```python
from build123d import *

# Parameters (mm, degrees)
SKETCH1_W           = 20
SKETCH1_H           = 20
BOSS_EXTRUDE1_DEPTH = 20
CUT_EXTRUDE1_DEPTH  = 20
CUT_EXTRUDE2_DEPTH  = 20
CUT_EXTRUDE3_DEPTH  = 20
CUT_EXTRUDE4_DEPTH  = 20


with BuildPart() as part:
    # Sketch1 → Boss-Extrude1 (new body)
    with BuildSketch(Plane.XY):
        with Locations((10, 10)):
            Rectangle(SKETCH1_W, SKETCH1_H)
    extrude(amount=BOSS_EXTRUDE1_DEPTH)

    # Sketch2 → Cut-Extrude1 (cut)
    with BuildSketch(Plane(origin=(0, 20, 0), x_dir=(1, 0, 0), z_dir=(0, 1, 0))):
        Polygon((20, 0), (10, 0), (20, -10), align=None)
    extrude(amount=-CUT_EXTRUDE1_DEPTH, mode=Mode.SUBTRACT)

    # Sketch3 → Cut-Extrude2 (cut)
    with BuildSketch(Plane(origin=(0, 20, 0), x_dir=(1, 0, 0), z_dir=(0, 1, 0))):
        Polygon((20, -20), (20, -10), (10, -20), align=None)
    extrude(amount=-CUT_EXTRUDE2_DEPTH, mode=Mode.SUBTRACT)

    # Sketch4 → Cut-Extrude3 (cut)
    with BuildSketch(Plane(origin=(0, 20, 0), x_dir=(1, 0, 0), z_dir=(0, 1, 0))):
        Polygon((0, 0), (10, 0), (0, -10), align=None)
    extrude(amount=-CUT_EXTRUDE3_DEPTH, mode=Mode.SUBTRACT)

    # Sketch5 → Cut-Extrude4 (cut)
    with BuildSketch(Plane(origin=(0, 20, 0), x_dir=(1, 0, 0), z_dir=(0, 1, 0))):
        Polygon((0, -20), (0, -10), (10, -20), align=None)
    extrude(amount=-CUT_EXTRUDE4_DEPTH, mode=Mode.SUBTRACT)


solid = part.part
```
Input: part model. Units: mm. Frame: model coordinates. Coordinates: 2 decimals unless noted, no trailing zeros. Write each loop counter-clockwise with the first axis right and the second up, starting at its lowest first coordinate (ties: lowest second). Pieces come first, ordered by that corner, then holes. Notation, with made-up numbers: (-13, -6.5) - (29, -6.5) arc R11 cw to (29, 14.5) - close; hole circle Ø10 at (0, 30.5). An arc over 180 degrees is marked (long way). Put each result on its own line as item: value. Start each with the question number.
1) Ray query, L1, parallel to Z at x = 3.25, y = 13.25; L2, parallel to X at y = 2.75, z = 17; L3, parallel to X at y = 19, z = 12.25. Return the intervals inside material, ascending.
2) Cut plane B-B (x = 4.25). Return the cut outline in (y, z), plus the area to 3 significant figures.
3) Contact query for flat-ended pins moving along their axis: pin 1 (3 mm diameter, centred on x = 14.5, y = 18, fed in from -Z); pin 2 (1.5 mm diameter, centred on y = 5.5, z = 17, fed in from -X); pin 3 (3 mm diameter, centred on y = 4, z = 3, fed in from -X). Output: stop coordinate, or through.
4) Cut plane A-A (z = 5). Return the cut outline in (x, y), plus the area to 3 significant figures.
Resolved:
1. L1: z = 6.75 to 13.25
1. L2: x = 7 to 13
1. L3: x = 2.25 to 17.75
2. outline: (0, 5.75) - (20, 5.75) - (20, 14.25) - (0, 14.25) - close
2. area: 170 mm2
3. pin 1: stops at z = 3
3. pin 2: stops at x = 6.25
3. pin 3: stops at x = 5.5
4. outline: (5, 0) - (15, 0) - (15, 20) - (5, 20) - close
4. area: 200 mm2
